from build123d import *

# Parameters (mm, degrees)
SKETCH1_W           = 152.4
SKETCH1_H           = 152.4
SKETCH1_R           = 64.135
BOSS_EXTRUDE1_DEPTH = 22.225
SKETCH2_W           = 152.4
SKETCH2_H           = 152.4
BOSS_EXTRUDE2_DEPTH = 76.2


with BuildPart() as part:
    # Sketch1 → Boss-Extrude1 (new body)
    with BuildSketch(Plane(origin=(0, 0, 0), x_dir=(1, 0, 0), z_dir=(0, 1, 0))):
        Rectangle(SKETCH1_W, SKETCH1_H)
        Circle(SKETCH1_R, mode=Mode.SUBTRACT)
    extrude(amount=BOSS_EXTRUDE1_DEPTH)

    # Sketch2 → Boss-Extrude2 (add)
    with BuildSketch(Plane(origin=(0, 0, 0), x_dir=(-1, 0, 0), z_dir=(0, -1, 0))):
        Rectangle(SKETCH2_W, SKETCH2_H)
    extrude(amount=BOSS_EXTRUDE2_DEPTH)


solid = part.part
Could you check a few things on this model? Use its own coordinates, in mm. A direction names the side the tool comes from. Give positions to 0.01 mm unless a question says otherwise; leave off trailing zeros. Order: outer loops, then holes, each group sorted by start corner. A loop starts at its lowest first (then second) coordinate and runs counter-clockwise, first axis right, second up. Notation, with made-up numbers: (7.25, 48) - (56.25, 48) arc R18 ccw to (56.25, 58) - close; hole circle Ø2 at (7, -23.75). An arc over 180 degrees is marked (long way). One line per question, with ' | ' between items. Start each with the question number.
Item 1: I'm going to push a flat-ended pin straight in: pin 1 Ø4 at (x, z) = (11.5, 39.5) entering from +Y. Where does the tip first touch, or does it pass through?
Item 2: I want a section at A-A on z = 0. Write out the boundary of the cut face in (x, y) (3 decimals), then the cut area to 3 significant figures.
Item 3: I want a section at B-B on y = 2. Write out the boundary of the cut face in (x, z) (3 decimals), then the cut area to 3 significant figures.
Item 4: Thinking about a two-plate mould opening in Z: for faces 3 (the flat face through (-76.2, -26, 1)), 4 (the flat face through (1, -26, -76.2)), 5 (the cylindrical face through (61.173, 10.957, -19.264)), which applies, pulls with the +Z half, pulls with the -Z half, needs draft (parallel to the pull), parting line crosses it, or undercut?
Item 5: For faces 1 (the flat face through (1, 0, -1)), 2 (the flat face through (1, -26, 76.2)), which set-ups out of +Z, -Z, +X, -X, +Y, -Y let a thin tool reach every point of the face, with its end or its side?
Item 6: I want a section at C-C on x = -20. Write out the boundary of the cut face in (y, z) (3 decimals).
Item 7: I need wall thicknesses on probe 1 along Z at (x, y) = (0, 10.25) (3 decimals); probe 2 along Y at (x, z) = (13, -39.5). Which ranges of each line are inside material? Lowest first, please. Write a range as [from, to].
Verdict:
1) pin 1: y = 0
2) outline: (-76.2, -76.2) - (76.2, -76.2) - (76.2, 22.225) - (64.135, 22.225) - (64.135, 0) - (-64.135, 0) - (-64.135, 22.225) - (-76.2, 22.225) - close | area: 12,100 mm^2
3) outline: (-76.2, -76.2) - (76.2, -76.2) - (76.2, 76.2) - (-76.2, 76.2) - close; hole circle Ø128.27 at (0, 0) | area: 10,300 mm^2
4) face 3: needs draft | face 4: pulls with the -Z half | face 5: undercut
5) face 1: +Y | face 2: +Z, +X, -X, +Y, -Y
6) outline: (-76.2, -76.2) - (22.225, -76.2) - (22.225, -60.937) - (0, -60.937) - (0, 60.937) - (22.225, 60.937) - (22.225, 76.2) - (-76.2, 76.2) - close
7) probe 1: [-76.2, -64.135], [64.135, 76.2] | probe 2: [-76.2, 0]
